Autodesk Inventor part; units mm, degrees
ref_plane "YZ Plane" through (0, 0, 0) normal (1, 0, 0) x (0, 1, 0)
ref_plane "XZ Plane" through (0, 0, 0) normal (0, 1, 0) x (-1, 0, 0)
ref_plane "XY Plane" through (0, 0, 0) normal (0, 0, 1) x (1, 0, 0)
sketch "Skizze1" plane through (0, 0, 0) normal (0, 0, 1) x (1, 0, 0)
  line L0 (-4.2, 0) -> (4.2, 0)
  line L1 (0, -4.2) -> (0, 4.2)
  line L2 (-3, 3) -> (3, 3)
  line L3 (3, 3) -> (3, -3)
  line L4 (3, -3) -> (-3, -3)
  line L5 (-3, -3) -> (-3, 3)
  point P0 (0, 0)
  dimension "d0" = 6
  dimension "d1" = 6
extrude "Extrusion1" add sketch "Skizze1" along normal blind 10
sketch "Skizze2" plane through (3, -3, 0) normal (1, 0, 0) x (0, 0, -1)
  line L0 (-10, 0) -> (-10, 6)
  line L1 (0, 0) -> (-10, 0)
  line L2 (-10, 6) -> (-6.5359, 0)
  point P0 (0, 3)
  dimension "d4" = 60
extrude "Extrusion2" cut sketch "Skizze2" against normal through all
fillet "Rundung1" radius 2 2 edges at (3, 0, 0) (-3, 0, 0)
sketch "Skizze3" plane through (0, 0, 0) normal (0, 0, -1) x (-1, 0, 0)
  point P0 (0, 0)
  point P1 (0, 0)
hole "Bohrung1" at (0, 0, 0) direction (0, 0, 1) diameter 2.459 end through all
hole "Bohrung2" at (0, 0, 0) direction (0, 0, 1) diameter 3.2 depth 1.5 tip angle 118
properties part number "13_1087_034"
Design review of the part built by this model. Coordinates are the model's own, in mm. A direction names the side the tool comes from. Coordinates: 2 decimals unless noted, no trailing zeros. Order: outer loops, then holes, each group sorted by start corner. A loop starts at its lowest first (then second) coordinate and runs counter-clockwise, first axis right, second up. Notation, with made-up numbers: M 2.5,81.25 L 48.5,81.25 A10 ccw 48.5,88.25 Z; hole C 69.25,7.5 d9. An arc over 180 degrees is marked long. Use a Markdown table: item, result.
(1) Add section D-D (y = 2.75). Give the boundary of the cut face in (x, z).
Worked answers:
| item | result |
|---|---|
| outline | M -3,2 A2 ccw -1,0 L 1,0 A2 ccw 3,2 L 3,9.86 L -3,9.86 Z |
(2) Wall thickness on probe 1 along X at (y, z) = (0, 4); probe 2 along Y at (x, z) = (0, 0.5): over which ranges is each line inside the solid? List them lowest first.
Worked answers:
| item | result |
|---|---|
| probe 1 | x = -3 to -1.23, 1.23 to 3 |
| probe 2 | y = -3 to -1.6, 1.6 to 3 |
(3) Add section B-B (x = 0). Give the boundary of the cut face in (y, z), then the cut area to 3 significant figures.
Worked answers:
| item | result |
|---|---|
| outline | M -3,0 L -1.6,0 L -1.6,1.5 L -1.23,1.72 L -1.23,7.56 L -3,6.54 Z; M 1.23,1.72 L 1.6,1.5 L 1.6,0 L 3,0 L 3,10 L 1.23,8.98 Z |
| area | 28.1 mm2 |
(4) For faces 1 (the cylindrical face through (-0.481, 1.526, 0.76)), 2 (the flat face through (0, -2, 0)), list the 3-axis set-ups (+Z, -Z, +X, -X, +Y, -Y) from which the entire face can be reached by the end or side of a thin tool; tool diameter is ignored.
Worked answers:
| item | result |
|---|---|
| face 1 | -Z |
| face 2 | -Z, +X, -X, +Y, -Y |
(5) Add section C-C (y = 0). Give the boundary of the cut face in (x, z), then the cut area to 3 significant figures.
Worked answers:
| item | result |
|---|---|
| outline | M -3,2 A2 ccw -1.6,0.09 L -1.6,1.5 L -1.23,1.72 L -1.23,8.27 L -3,8.27 Z; M 1.23,1.72 L 1.6,1.5 L 1.6,0.09 A2 ccw 3,2 L 3,8.27 L 1.23,8.27 Z |
| area | 26.4 mm2 |
(6) For P1, Ø1.5, axis at x = 1.5, y = 2, coming from the +Z side; P2, Ø3, axis at x = 0, y = 0, coming from the +Z side, all flat-tipped, find the tip position at first contact; note any pin that passes through.
Worked answers:
| item | result |
|---|---|
| P1 | stops at z = 9.86 |
| P2 | stops at z = 9.13 |
(7) Draft analysis for pull direction Y (two halves, no side actions). For faces 3 (the cylindrical face through (-0.369, 1.173, 5.401)), 4 (the flat face through (0, 3, 5)), 5 (the flat face through (1.38, 0.04, 8.29)), 6 (the flat face through (3, 0, 5)), state which applies: released by +Y, released by -Y, zero draft, split by the parting line, or undercut.
Worked answers:
| item | result |
|---|---|
| face 3 | undercut |
| face 4 | released by +Y |
| face 5 | released by -Y |
| face 6 | zero draft |
(8) Add section A-A (z = 3.25). Give the boundary of the cut face in (x, y), then the cut area to 3 significant figures.
Worked answers:
| item | result |
|---|---|
| outline | M -3,-3 L 3,-3 L 3,3 L -3,3 Z; hole C 0,0 d2.46 |
| area | 31.3 mm2 |
